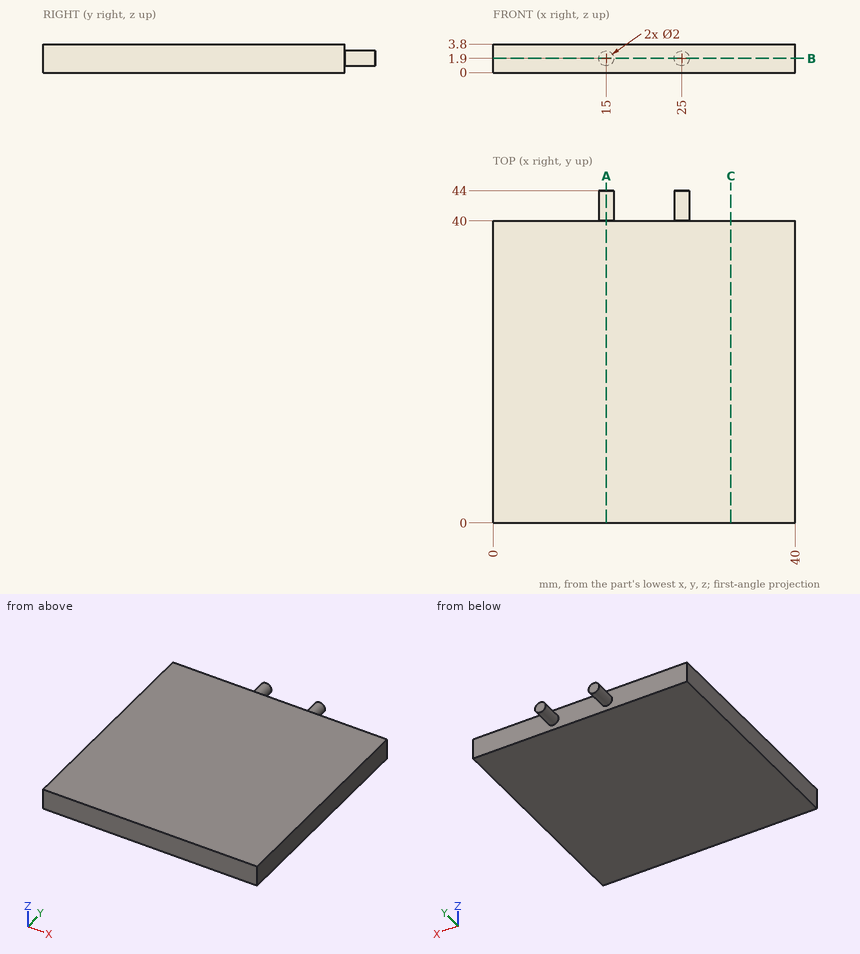
Can you work these out from the drawing? Everything is in mm from the part's minimum corner. Give positions to 0.01 mm unless a question says otherwise; leave off trailing zeros. Write each loop counter-clockwise with the first axis right and the second up, starting at its lowest first coordinate (ties: lowest second). Pieces come first, ordered by that corner, then holes. Notation, with made-up numbers: M -8,54 L 13,54 A29 ccw 13,82 Z; hole C -2.5,24 d8. An arc over 180 degrees is marked long. Answer in a Markdown table with one row per item. Add a question column.
Item 1: For pin 1 Ø1.1 at (x, z) = (30, 1.5) entering from +Y, with a flat end and sliding along its axis, tell me the tip position at first contact or that it passes through.
Item 2: Please list where this line runs through material, in increasing order: L1, parallel to Y at x = 4, z = 3.65.
Item 3: Imagine slicing it at C-C, the plane x = 31.5. Write out the boundary of the cut face in (y, z).
Item 4: Imagine slicing it at A-A, the plane x = 15. Write out the boundary of the cut face in (y, z), plus the area to 3 significant figures.
Item 5: Imagine slicing it at B-B, the plane z = 1.9. Write out the boundary of the cut face in (x, y).
Evaluation:
| question | item | result |
|---|---|---|
| 1 | pin 1 | stops at y = 40 |
| 2 | L1 | y = 0 to 40 |
| 3 | outline | M 0,0 L 40,0 L 40,3.8 L 0,3.8 Z |
| 4 | outline | M 0,0 L 40,0 L 40,0.9 L 44,0.9 L 44,2.9 L 40,2.9 L 40,3.8 L 0,3.8 Z |
| 4 | area | 160 mm² |
| 5 | outline | M 0,0 L 40,0 L 40,40 L 26,40 L 26,44 L 24,44 L 24,40 L 16,40 L 16,44 L 14,44 L 14,40 L 0,40 Z |
